Read the model definition and answer for the solid it produces. Units are mm, in the model's axes. Round coordinates to 2 decimals unless told otherwise and drop trailing zeros. Write each loop counter-clockwise with the first axis right and the second up, starting at its lowest first coordinate (ties: lowest second). Pieces come first, ordered by that corner, then holes. Notation, with made-up numbers: (-5.75, 14) -> (31.25, 14) arc R18 cw to (31.25, 29) -> close; hole circle Ø9 at (54, 0.5). An arc over 180 degrees is marked (long way). Return JSON: item names as keys, results as strings. Group by question number.
(1) A cutting plane is placed at B-B on x = -21.5. Give the vertices of the cut face in (y, z), then the cut area to 3 significant figures.
(2) A cutting plane is placed at D-D on z = -10.5. Give the vertices of the cut face in (x, y), then the cut area to 3 significant figures.
(3) Given pin 1 (3 mm diameter, centred on y = 5.5, z = -53, fed in from +X); pin 2 (3.5 mm diameter, centred on x = -55, y = 4, fed in from +Z); pin 3 (2.5 mm diameter, centred on x = -8, y = 4, fed in from +Z), each flat-ended and moving along its own axis, determine where each tip first touches the part or whether it passes through.
(4) Straight lines are drawn through the part: line 1 (X direction, y = 5.75, z = -17.5); line 2 (X direction, y = 4, z = -53); line 3 (Z direction, x = -21.5, y = 6.25). For each, find the intervals that lie inside material, in ascending order.
(5) A cutting plane is placed at C-C on y = 7. Give the vertices of the cut face in (x, z).
(6) A cutting plane is placed at A-A on z = -17.5. Give the vertices of the cut face in (x, y), then the cut area to 3 significant figures.
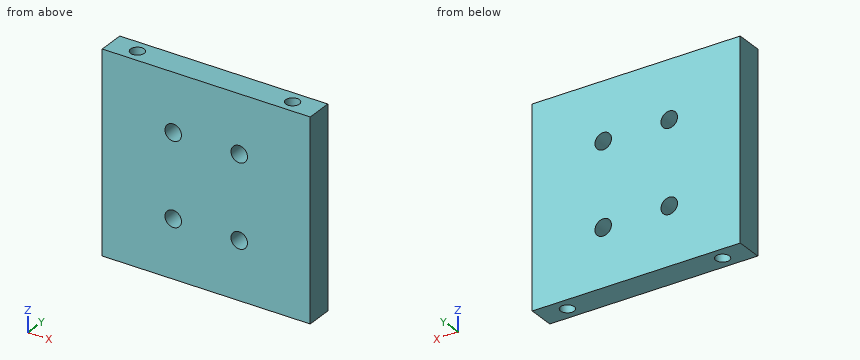
Autodesk Inventor part; units mm, degrees
ref_plane "YZ Plane" through (0, 0, 0) normal (1, 0, 0) x (0, 1, 0)
ref_plane "XZ Plane" through (0, 0, 0) normal (0, 1, 0) x (-1, 0, 0)
ref_plane "XY Plane" through (0, 0, 0) normal (0, 0, 1) x (1, 0, 0)
sketch "Sketch5" plane through (0, 0, 0) normal (0, 1, 0) x (-1, 0, 0)
  line L0 (0, 0) -> (63, 0)
  line L1 (63, 0) -> (63, -60)
  line L2 (63, -60) -> (0, -60)
  line L3 (0, -60) -> (0, 0)
  dimension "d68" = 63
  dimension "d69" = 60
extrude "Extrusion2" add sketch "Sketch5" along normal blind 8
sketch "Sketch6" plane through (0, 8, 0) normal (0, 1, 0) x (1, 0, 0)
  line L0 (-63, 60) -> (-63, 0)
  line L1 (0, 60) -> (-63, 60)
  point P0 (0, 0)
  point P1 (-41.5, 42.5)
  point P2 (-41.5, 17.5)
  point P3 (-21.5, 42.5)
  point P4 (-21.5, 17.5)
  dimension "d74" = 25
  dimension "d77" = 20
  dimension "d80" = 63
  dimension "d81" = 60
  dimension "d82" = 21.5
  dimension "d83" = 17.5
hole "Hole3" at (-41.5, 8, -42.5) at (-41.5, 8, -17.5) at (-21.5, 8, -42.5) at (-21.5, 8, -17.5) direction (0, -1, 0) diameter 5 end through all
sketch "Sketch7" plane through (-63, 0, 0) normal (0, 0, 1) x (1, 0, 0)
  line L0 (0, 0) -> (0, 8)
  line L1 (63, 0) -> (63, 8)
  point P0 (55, 4)
  point P1 (8, 4)
  point P2 (0, 4)
  dimension "d91" = 8
  dimension "d92" = 8
hole "Hole4" at (-8, 4, 0) at (-55, 4, 0) direction (0, 0, -1) diameter 4.134 depth 14.2 tip angle 118
sketch "Sketch8" plane through (0, 0, -60) normal (0, 0, -1) x (-1, 0, 0)
  circle A0 centre (8, 4) radius 2.067
  circle A1 centre (55, 4) radius 2.067
  point P0 (0, 0)
hole "Hole5" at (-8, 4, -60) at (-55, 4, -60) direction (0, 0, 1) diameter 4.134 depth 14.2 tip angle 118
equation "\"d89\" = Thickness"
equation "\"BendRadius\" = Thickness"
equation "\"BendReliefWidth\" = Thickness"
equation "\"BendReliefDepth\" = 0.5 * Thickness"
equation "\"TransitionRadius\" = BendRadius"
equation "\"JacobiRadiusSize\" = BendRadius"
equation "\"GapSize\" = Thickness"
properties part number "Traseira da caixa de sustentação" material "Aluminum 6061"
Checks:
{
 "1": {"outline": "(0, -60) -> (8, -60) -> (8, -45) -> (0, -45) -> close; (0, -40) -> (8, -40) -> (8, -20) -> (0, -20) -> close; (0, -15) -> (8, -15) -> (8, 0) -> (0, 0) -> close", "area": "400 mm^2"},
 "2": {"outline": "(-63, 0) -> (0, 0) -> (0, 8) -> (-63, 8) -> close; hole circle Ø4.13 at (-55, 4); hole circle Ø4.13 at (-8, 4)", "area": "477 mm^2"},
 "3": {"pin 1": "stops at x = 0", "pin 2": "stops at z = -14.39", "pin 3": "stops at z = -14.69"},
 "4": {"line 1": "x = -63 to -44, -39 to -24, -19 to 0", "line 2": "x = -63 to -57.07, -52.93 to -10.07, -5.93 to 0", "line 3": "z = -60 to -45, -40 to -20, -15 to 0"},
 "5": {"outline": "(-63, -60) -> (0, -60) -> (0, 0) -> (-63, 0) -> close; hole circle Ø5 at (-41.5, -42.5); hole circle Ø5 at (-41.5, -17.5); hole circle Ø5 at (-21.5, -42.5); hole circle Ø5 at (-21.5, -17.5)"},
 "6": {"outline": "(-63, 0) -> (-44, 0) -> (-44, 8) -> (-63, 8) -> close; (-39, 0) -> (-24, 0) -> (-24, 8) -> (-39, 8) -> close; (-19, 0) -> (0, 0) -> (0, 8) -> (-19, 8) -> close", "area": "424 mm^2"}
}
